Can you work these out from the model? Positions are in its coordinate system, mm. Face numbers are marked on the shaded views. A direction names the side the tool comes from. Coordinates: 2 decimals unless noted, no trailing zeros. Order: outer loops, then holes, each group sorted by start corner. A loop starts at its lowest first (then second) coordinate and runs counter-clockwise, first axis right, second up. Notation, with made-up numbers: (86.25, 34.5) -> (130.25, 34.5) arc R23 cw to (130.25, 64.5) -> close; hole circle Ø2 at (15.25, -25). An arc over 180 degrees is marked (long way). Use a Markdown table: item, result. Add a question column.
1. Suppose I cut it at B-B, the plane y = 46. List the corners of the cut face in (x, z) for me, then the cut area to 3 significant figures.
2. For the marked faces 4, 5 and 6, which set-ups out of +Z, -Z, +X, -X, +Y, -Y let a thin tool reach every point of the face, with its end or its side?
3. For pin 1 Ø1.5 at (x, y) = (7, 46.5) entering from -Z; pin 2 Ø2 at (x, y) = (-4.5, 43.5) entering from -Z; pin 3 Ø1 at (y, z) = (43.5, 9) entering from -X; pin 4 Ø3.5 at (y, z) = (45.5, 0) entering from -X, each with a flat end and sliding along its axis, tell me the tip position at first contact or that it passes through.
4. Suppose I cut it at A-A, the plane x = 0. List the corners of the cut face in (y, z) for me (3 decimals).
5. Suppose I cut it at C-C, the plane z = 0. State how many separate pieces and enclosed holes the cut face has, then the cut area to 3 significant figures.
6. If I drill on line 1 along Y through (x, z) = (3.85, 0); line 2 along Y through (x, z) = (5, 0); line 3 along X through (y, z) = (38, 0) (3 decimals), over which ranges is the centre line in solid material (lowest first)? Write a range as from..to.
7. Suppose I cut it at D-D, the plane x = 5. List the corners of the cut face in (y, z) for me, then the cut area to 3 significant figures.
8. We'd pull the mould along X, two halves only. Please class the marked faces 1, 2 and 3: pulls with the +X half, pulls with the -X half, needs draft (parallel to the pull), parting line crosses it, or undercut.
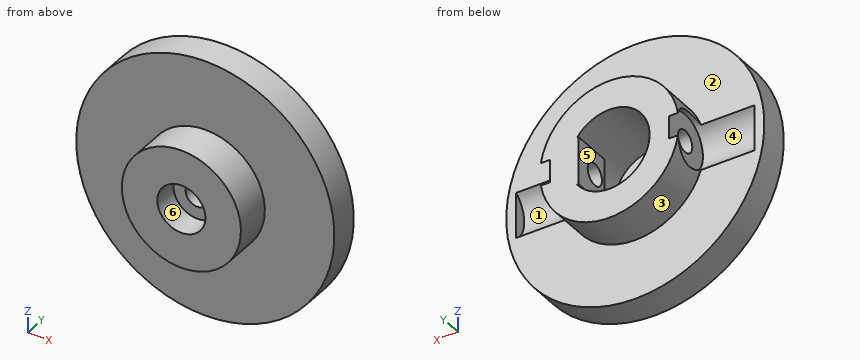
```python
from build123d import *

# Parameters (mm, degrees)
STOCK_HORN_DRIVE_FLANGE_START                 = 41
STOCK_HORN_DRIVE_FLANGE_PROFILE_R             = 13
STOCK_HORN_DRIVE_FLANGE_PROFILE_R_2           = 4.05
STOCK_HORN_DRIVE_FLANGE_DEPTH                 = 3
D_COUPLING_RING_START                         = 44
D_COUPLING_RING_PROFILE_R                     = 7
D_COUPLING_RING_PROFILE_R_2                   = 4.05
D_COUPLING_RING_DEPTH                         = 4
D_KEY_LAND_START                              = 44
D_KEY_LAND_PROFILE_W                          = 2.9
D_KEY_LAND_PROFILE_H                          = 4.8
D_KEY_LAND_DEPTH                              = 4
YAW_POSITIVE_RETENTION_CROSSBOLT_START        = -10
YAW_POSITIVE_RETENTION_CROSSBOLT_PROFILE_R    = 1.1
YAW_POSITIVE_RETENTION_CROSSBOLT_DEPTH        = 62.400389104
CROSSBOLT_FLAT_SEAT_CUT_12_START              = -12
CROSSBOLT_FLAT_SEAT_12_R                      = 2.75
CROSSBOLT_FLAT_SEAT_CUT_12_DEPTH              = 6
CROSSBOLT_FLAT_SEAT_CUT_6_START               = 6
CROSSBOLT_FLAT_SEAT_6_R                       = 2.75
CROSSBOLT_FLAT_SEAT_CUT_6_DEPTH               = 6
SG90_SPLINE_SOCKET_BOSS_OD12_START            = 37.3
SG90_SPLINE_SOCKET_BOSS_PROFILE_R             = 6
SG90_SPLINE_SOCKET_BOSS_OD12_DEPTH            = 3.7
SG90_SPLINE_PRESS_SOCKET_D4P85_DEPTH2P5_START = 37.3
SG90_SPLINE_PRESS_SOCKET_D4P85_DEPTH_2_R      = 2.425
SG90_SPLINE_PRESS_SOCKET_D4P85_DEPTH2P5_DEPTH = 2.5
SG90_CENTRE_SCREW_CLEARANCE_D2P4_START        = 39.8
SG90_CENTRE_SCREW_CLEARANCE_D2P4_PROFILE_R    = 1.2
SG90_CENTRE_SCREW_CLEARANCE_D2P4_DEPTH        = 1.2


with BuildPart() as part:
    # Stock_horn_drive_flange_profile → Stock_horn_drive_flange (new body)
    with BuildSketch(Plane(origin=(0, 0, 0), x_dir=(1, 0, 0), z_dir=(0, 1, 0)).offset(STOCK_HORN_DRIVE_FLANGE_START)):
        with Locations(Location((0, 0, 0), (0, 0, 270))):
            Circle(STOCK_HORN_DRIVE_FLANGE_PROFILE_R)
        with Locations(Location((0, 0, 0), (0, 0, 270))):
            Circle(STOCK_HORN_DRIVE_FLANGE_PROFILE_R_2, mode=Mode.SUBTRACT)
    extrude(amount=STOCK_HORN_DRIVE_FLANGE_DEPTH)

    # D_coupling_ring_profile → D_coupling_ring (add)
    with BuildSketch(Plane(origin=(0, 0, 0), x_dir=(1, 0, 0), z_dir=(0, 1, 0)).offset(D_COUPLING_RING_START)):
        with Locations(Location((0, 0, 0), (0, 0, 270))):
            Circle(D_COUPLING_RING_PROFILE_R)
        with Locations(Location((0, 0, 0), (0, 0, 270))):
            Circle(D_COUPLING_RING_PROFILE_R_2, mode=Mode.SUBTRACT)
    extrude(amount=D_COUPLING_RING_DEPTH)

    # D_key_land_profile → D_key_land (add)
    with BuildSketch(Plane(origin=(0, 0, 0), x_dir=(1, 0, 0), z_dir=(0, 1, 0)).offset(D_KEY_LAND_START)):
        with Locations((4.55, 0)):
            Rectangle(D_KEY_LAND_PROFILE_W, D_KEY_LAND_PROFILE_H)
    extrude(amount=D_KEY_LAND_DEPTH)

    # Yaw_positive_retention_crossbolt_profile → Yaw_positive_retention_crossbolt (cut, through all)
    with BuildSketch(Plane(origin=(0, 0, 0), x_dir=(0, 0, -1), z_dir=(1, 0, 0)).offset(YAW_POSITIVE_RETENTION_CROSSBOLT_START)):
        with Locations(Location((0, 45.5, 0), (0, 0, 180))):
            Circle(YAW_POSITIVE_RETENTION_CROSSBOLT_PROFILE_R)
    extrude(amount=YAW_POSITIVE_RETENTION_CROSSBOLT_DEPTH, mode=Mode.SUBTRACT)

    # Crossbolt_flat_seat_-12 → Crossbolt_flat_seat_cut_-12 (cut)
    with BuildSketch(Plane(origin=(0, 0, 0), x_dir=(0, 0, -1), z_dir=(1, 0, 0)).offset(CROSSBOLT_FLAT_SEAT_CUT_12_START)):
        with Locations((0, 45.5)):
            Circle(CROSSBOLT_FLAT_SEAT_12_R)
    extrude(amount=CROSSBOLT_FLAT_SEAT_CUT_12_DEPTH, mode=Mode.SUBTRACT)

    # Crossbolt_flat_seat_6 → Crossbolt_flat_seat_cut_6 (cut)
    with BuildSketch(Plane(origin=(0, 0, 0), x_dir=(0, 0, -1), z_dir=(1, 0, 0)).offset(CROSSBOLT_FLAT_SEAT_CUT_6_START)):
        with Locations((0, 45.5)):
            Circle(CROSSBOLT_FLAT_SEAT_6_R)
    extrude(amount=CROSSBOLT_FLAT_SEAT_CUT_6_DEPTH, mode=Mode.SUBTRACT)

    # SG90_spline_socket_boss_profile → SG90_spline_socket_boss_OD12 (add)
    with BuildSketch(Plane(origin=(0, 0, 0), x_dir=(1, 0, 0), z_dir=(0, 1, 0)).offset(SG90_SPLINE_SOCKET_BOSS_OD12_START)):
        with Locations(Location((0, 0, 0), (0, 0, 270))):
            Circle(SG90_SPLINE_SOCKET_BOSS_PROFILE_R)
    extrude(amount=SG90_SPLINE_SOCKET_BOSS_OD12_DEPTH)

    # SG90_spline_press_socket_D4p85_depth 2 → SG90_spline_press_socket_D4p85_depth2p5 (cut)
    with BuildSketch(Plane(origin=(0, 0, 0), x_dir=(1, 0, 0), z_dir=(0, 1, 0)).offset(SG90_SPLINE_PRESS_SOCKET_D4P85_DEPTH2P5_START)):
        with Locations(Location((0, 0, 0), (0, 0, 270))):
            Circle(SG90_SPLINE_PRESS_SOCKET_D4P85_DEPTH_2_R)
    extrude(amount=SG90_SPLINE_PRESS_SOCKET_D4P85_DEPTH2P5_DEPTH, mode=Mode.SUBTRACT)

    # SG90_centre_screw_clearance_D2p4_profile → SG90_centre_screw_clearance_D2p4 (cut)
    with BuildSketch(Plane(origin=(0, 0, 0), x_dir=(1, 0, 0), z_dir=(0, 1, 0)).offset(SG90_CENTRE_SCREW_CLEARANCE_D2P4_START)):
        with Locations(Location((0, 0, 0), (0, 0, 270))):
            Circle(SG90_CENTRE_SCREW_CLEARANCE_D2P4_PROFILE_R)
    extrude(amount=SG90_CENTRE_SCREW_CLEARANCE_D2P4_DEPTH, mode=Mode.SUBTRACT)


solid = part.part
```
Worked out:
| question | item | result |
|---|---|---|
| 1 | outline | (-6.46, -2.7) arc R7 ccw to (6.46, -2.7) -> (6, -2.7) -> (6, -0.98) -> (3.1, -0.98) -> (3.1, -2.4) -> (3.26, -2.4) arc R4.05 cw to (-3.93, -0.98) -> (-6, -0.98) -> (-6, -2.7) -> close; (-6.46, 2.7) -> (-6, 2.7) -> (-6, 0.98) -> (-3.93, 0.98) arc R4.05 cw to (3.26, 2.4) -> (3.1, 2.4) -> (3.1, 0.98) -> (6, 0.98) -> (6, 2.7) -> (6.46, 2.7) arc R7 ccw to start |
| 1 | area | 87.3 mm² |
| 2 | face 4 | none |
| 2 | face 5 | +Y |
| 2 | face 6 | -Y |
| 3 | pin 1 | stops at z = -3.15 |
| 3 | pin 2 | stops at z = -12.52 |
| 3 | pin 3 | stops at x = -9.84 |
| 3 | pin 4 | stops at x = -13 |
| 4 | outline | (37.3, -6) -> (41, -6) -> (41, -13) -> (44, -13) -> (44, -7) -> (48, -7) -> (48, -4.05) -> (41, -4.05) -> (41, -1.2) -> (39.8, -1.2) -> (39.8, -2.425) -> (37.3, -2.425) -> close; (37.3, 2.425) -> (39.8, 2.425) -> (39.8, 1.2) -> (41, 1.2) -> (41, 4.05) -> (48, 4.05) -> (48, 7) -> (44, 7) -> (44, 13) -> (41, 13) -> (41, 6) -> (37.3, 6) -> close |
| 5 | separate pieces | 4 |
| 5 | enclosed holes | 0 |
| 5 | area | 76.8 mm² |
| 6 | line 1 | y = 37.3..41, 44..44.4, 46.6..48 |
| 6 | line 2 | y = 37.3..44.4, 46.6..48 |
| 6 | line 3 | x = -6..-2.425, 2.425..6 |
| 7 | outline | (37.3, -3.32) -> (41, -3.32) -> (41, -12) -> (44, -12) -> (44, -4.9) -> (48, -4.9) -> (48, 4.9) -> (44, 4.9) -> (44, 12) -> (41, 12) -> (41, 3.32) -> (37.3, 3.32) -> close; hole circle Ø2.2 at (45.5, 0) |
| 7 | area | 132 mm² |
| 8 | face 1 | undercut |
| 8 | face 2 | needs draft |
| 8 | face 3 | parting line crosses it |
